Part print with two shaded views. Sizes in mm from the minimum x, y, z corner. A direction names the side the tool comes from. Round coordinates to 2 decimals unless told otherwise and drop trailing zeros. Loops run counter-clockwise (first coordinate to the right, second up) from the corner with the lowest first, then second, coordinate; pieces in that order, holes last. Notation, with made-up numbers: M 41.25,16.5 L 97.25,16.5 A28 cw 97.25,53.5 Z; hole C 85.25,3.5 d10. An arc over 180 degrees is marked long. Use a Markdown table: item, result. Add a question column.
Item 1: Saw through at A-A on x = 30. Write the cut outline in (y, z), then the cut area to 3 significant figures.
Item 2: Tool access for the marked faces 4 and 5: list every direction of +Z, -Z, +X, -X, +Y, -Y with a clear straight run to the whole face (end or side of a thin tool).
Item 3: Wall check: L1, parallel to Y at x = 30, z = 7; L2, parallel to Y at x = 28, z = 2.75; L3, parallel to Y at x = 26.5, z = 6. Give the ranges that are in metal, low to high. Write a range as from..to.
Item 4: Pin check, flat tips, straight feed: P1, Ø1, axis at y = 20, z = 6.5, coming from the +X side; P2, Ø1, axis at y = 44, z = 2, coming from the -X side; P3, Ø2, axis at x = 44, z = 7.5, coming from the -Y side; P4, Ø6.5, axis at x = 30, y = 30, coming from the +Z side. Stop position of each tip, or through.
Item 5: Saw through at C-C on z = 15.75. Write the cut outline in (x, y).
Item 6: Two-plate mould, pull along X, no slides. Class the marked faces 1, 2 and 3: +X half, -X half, draft (parallel to the pull), parting line (faces both ways), or undercut.
Item 7: Saw through at D-D on z = 7. Write the cut outline in (x, y), then the cut area to 3 significant figures.
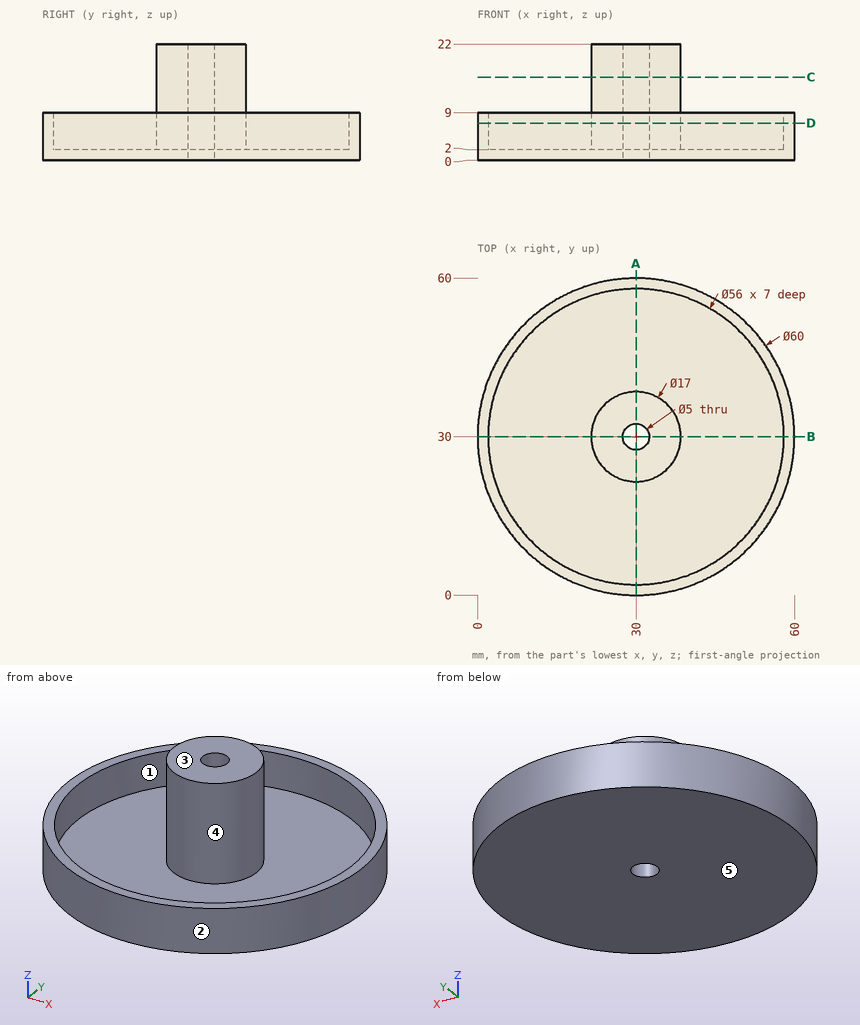
Entries:
| question | item | result |
|---|---|---|
| 1 | outline | M 0,0 L 27.5,0 L 27.5,22 L 21.5,22 L 21.5,2 L 2,2 L 2,9 L 0,9 Z; M 32.5,0 L 60,0 L 60,9 L 58,9 L 58,2 L 38.5,2 L 38.5,22 L 32.5,22 Z |
| 1 | area | 378 mm2 |
| 2 | face 4 | +Z |
| 2 | face 5 | -Z, +X, -X, +Y, -Y |
| 3 | L1 | 0..2, 21.5..27.5, 32.5..38.5, 58..60 |
| 3 | L2 | 0.07..2.07, 21.74..28.5, 31.5..38.26, 57.93..59.93 |
| 3 | L3 | 0.2..2.22, 22.25..37.75, 57.78..59.8 |
| 4 | P1 | x = 58.46 |
| 4 | P2 | x = 3.21 |
| 4 | P3 | y = 2.96 |
| 4 | P4 | z = 22 |
| 5 | outline | C 30,30 d17; hole C 30,30 d5 |
| 6 | face 1 | undercut |
| 6 | face 2 | parting line |
| 6 | face 3 | draft |
| 7 | outline | C 30,30 d60; C 30,30 d17; hole C 30,30 d56; hole C 30,30 d5 |
| 7 | area | 572 mm2 |
